Verification items for this drawing (mm, ordinates from the low corner). A direction names the side the tool comes from. Coordinates: 2 decimals unless noted, no trailing zeros. Order: outer loops, then holes, each group sorted by start corner. A loop starts at its lowest first (then second) coordinate and runs counter-clockwise, first axis right, second up. Notation, with made-up numbers: (68.5, -30.5) -> (77.5, -30.5) arc R16 ccw to (77.5, 0.5) -> close; hole circle Ø9 at (69.25, -21.75). An arc over 180 degrees is marked (long way). Answer as CSV lines item,"result". Start each with the question number.
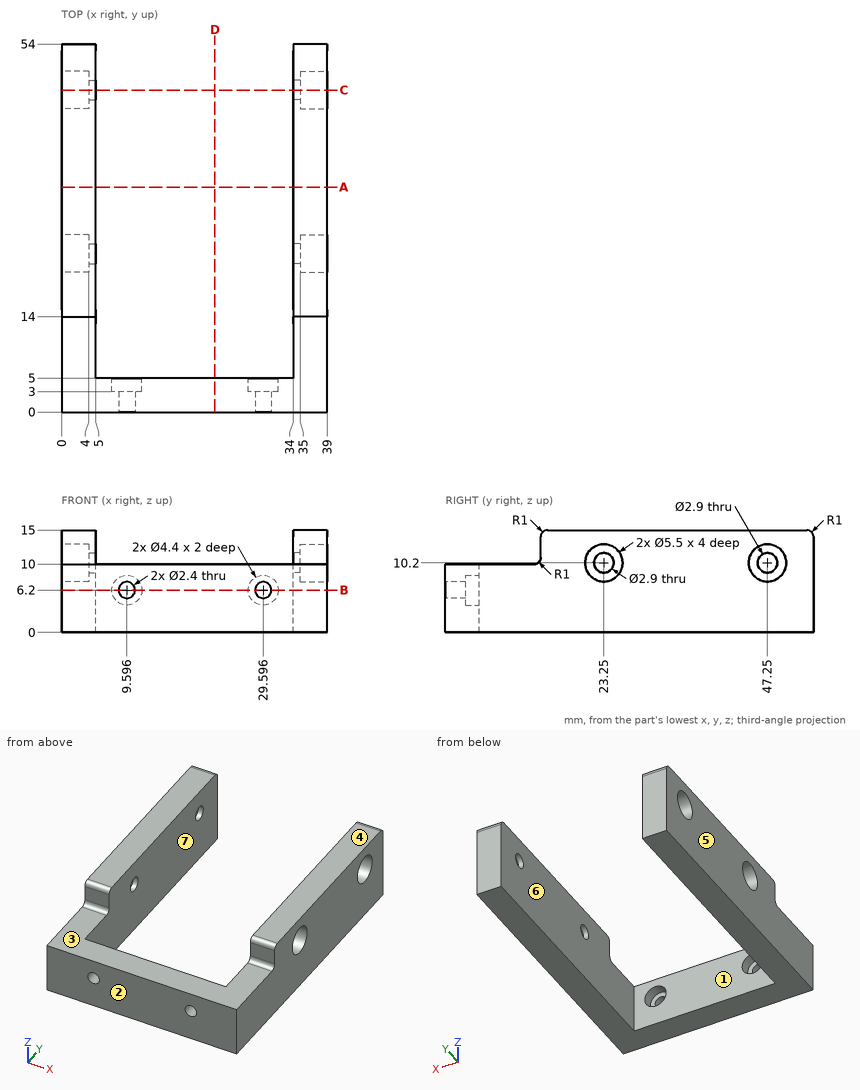
Q1. Release check for a two-part mould opening along X. For the marked faces 4, 5, 6 and 7 record: released by +X, released by -X, zero draft, split by the parting line, or undercut.
Q2. Sectioned sample at C-C, the plane y = 47.25. Record the cut outline in (x, z), then the cut area to 3 significant figures.
Q3. Sectioned sample at D-D, the plane x = 22.5. Record the cut outline in (y, z), then the cut area to 3 significant figures.
Q4. Access from +Z, -Z, +X, -X, +Y, -Y to the whole of each face (thin tool, end or side, straight path). Record for the marked faces 1, 2 and 3.
Q5. Thickness scan on L1, parallel to X at y = 12, z = 9; L2, parallel to Y at x = 1.9, z = 10.2; L3, parallel to Y at x = 34.2, z = 10.2. Record the ranges inside material, lowest first.
Q6. Go/stop test with flat-tipped pins: pin 1 Ø3 at (y, z) = (23.5, 11) entering from -X; pin 2 Ø5 at (x, z) = (16.5, 2.5) entering from +Y; pin 3 Ø1.5 at (x, z) = (37, 12) entering from -Y; pin 4 Ø6 at (y, z) = (48, 11) entering from +X. Record where each tip stops, or that it passes through.
Q7. Sectioned sample at B-B, the plane z = 6.2. Record the cut outline in (x, y) (1 decimal).
Q8. Sectioned sample at A-A, the plane y = 33. Record the cut outline in (x, z).
Geometry results:
1,face 4,"zero draft"
1,face 5,"released by -X"
1,face 6,"undercut"
1,face 7,"undercut"
2,outline,"(0, 0) -> (5, 0) -> (5, 8.75) -> (4, 8.75) -> (4, 7.45) -> (0, 7.45) -> close; (0, 12.95) -> (4, 12.95) -> (4, 11.65) -> (5, 11.65) -> (5, 15) -> (0, 15) -> close; (34, 0) -> (39, 0) -> (39, 7.45) -> (35, 7.45) -> (35, 8.75) -> (34, 8.75) -> close; (34, 11.65) -> (35, 11.65) -> (35, 12.95) -> (39, 12.95) -> (39, 15) -> (34, 15) -> close"
2,area,"100 mm^2"
3,outline,"(0, 0) -> (5, 0) -> (5, 10) -> (0, 10) -> close"
3,area,"50.0 mm^2"
4,face 1,"+Z, -Z, +Y"
4,face 2,"+Z, -Z, +X, -X, -Y"
4,face 3,"+Z, +X, -X, -Y"
5,L1,"x = 0 to 5, 34 to 39"
5,L2,"y = 13.6 to 20.5, 26 to 44.5, 50 to 54"
5,L3,"y = 13.6 to 21.8, 24.7 to 45.8, 48.7 to 54"
6,pin 1,"stops at x = 4"
6,pin 2,"stops at y = 5"
6,pin 3,"stops at y = 14"
6,pin 4,"stops at x = 39"
7,outline,"(0, 0) -> (8.4, 0) -> (8.4, 3) -> (7.4, 3) -> (7.4, 5) -> (5, 5) -> (5, 54) -> (0, 54) -> close; (10.8, 0) -> (28.4, 0) -> (28.4, 3) -> (27.4, 3) -> (27.4, 5) -> (11.8, 5) -> (11.8, 3) -> (10.8, 3) -> close; (30.8, 0) -> (39, 0) -> (39, 54) -> (34, 54) -> (34, 5) -> (31.8, 5) -> (31.8, 3) -> (30.8, 3) -> close"
8,outline,"(0, 0) -> (5, 0) -> (5, 15) -> (0, 15) -> close; (34, 0) -> (39, 0) -> (39, 15) -> (34, 15) -> close"
